```python
from build123d import *

# Parameters (mm, degrees)
F0_R      = 3
F0_R_2    = 2
F1_DEPTH  = 100
F2_R      = 3
F2_R_2    = 2
F3_DEPTH  = 6
F4_W      = 2
F4_H      = 7
F6_DEPTH  = 12.5
F5_W      = 2
F5_H      = 7
F7_DEPTH  = 12.5
F8_R      = 2
F9_DEPTH  = 34
F10_R     = 3.5
F10_R_2   = 3
F10_R_3   = 2
F11_DEPTH = 3


# Not quite as in the source:
# - a fillet or chamfer that OpenCascade refuses, or shapes differently, is made with other operations: its cross-section is extruded or revolved along the edge and cut away or added


with BuildPart() as f1:
    # F0 (on Top) → F1 (new body)
    with BuildSketch(Plane.XY):
        Circle(F0_R)
        Circle(F0_R_2, mode=Mode.SUBTRACT)
    extrude(amount=F1_DEPTH)

    # F2 (on face) → F3 (join)
    with BuildSketch(Plane.XY.offset(100)):
        Circle(F2_R)
        Circle(F2_R_2, mode=Mode.SUBTRACT)
        Circle(F2_R_2)
    extrude(amount=F3_DEPTH)

    # F4 (on Front) → F6 (cut, symmetric)
    with BuildSketch(Plane.XZ):
        with Locations((0, 85.1259604096)):
            Rectangle(F4_W, F4_H)
    extrude(amount=F6_DEPTH, both=True, mode=Mode.SUBTRACT)

    # F5 (on Right) → F7 (cut, symmetric)
    with BuildSketch(Plane.YZ):
        with Locations((0, 94.9563682079)):
            Rectangle(F5_W, F5_H)
    extrude(amount=F7_DEPTH, both=True, mode=Mode.SUBTRACT)

    # F8
    f8_edges = [f1.edges().sort_by_distance(p)[0] for p in [
        (-3, 0, 106),
    ]]
    fillet(f8_edges, radius=F8_R)

    # F9 (add): a face of the model
    f9_faces = [f1.faces().sort_by_distance(p)[0] for p in [
        (-2.9151471863, 0, 0),
    ]]
    extrude(f9_faces, amount=F9_DEPTH)

    # F10 (on face) → F11 (join)
    with BuildSketch(Plane(origin=(0, 0, -34), x_dir=(1, 0, 0), z_dir=(0, 0, -1))):
        Circle(F10_R)
        Circle(F10_R_2, mode=Mode.SUBTRACT)
        Circle(F10_R_2)
        Circle(F10_R_3, mode=Mode.SUBTRACT)
    extrude(amount=F11_DEPTH)

    # F12: fillet of radius 1 on 2 edges, made by hand

    # F12_s1 → F12_t2 (revolve, cut)
    with BuildSketch(Plane.XZ):
        with BuildLine():
            ThreePointArc((3, -34), (3.3660254038, -34.3660254038), (3.5, -34.8660254038))
            Line((3.5, -34.8660254038), (3.5, -34))
            Line((3.5, -34), (3, -34))
        make_face()
    revolve(axis=Axis((0, 0, -34), (0, 0, -1)), mode=Mode.SUBTRACT)

    # F12_s3 → F12_t4 (revolve, cut)
    with BuildSketch(Plane.XZ):
        with BuildLine():
            ThreePointArc((3.5, -36), (3.2071067812, -36.7071067812), (2.5, -37))
            Line((2.5, -37), (3.5, -37))
            Line((3.5, -37), (3.5, -36))
        make_face()
    revolve(axis=Axis((0, 0, -37), (0, 0, -1)), mode=Mode.SUBTRACT)


solid = f1.part
```
The model under review builds one solid part; all positions refer to its coordinate system, in mm. Round coordinates to 2 decimals unless told otherwise and drop trailing zeros. Loops run counter-clockwise (first coordinate to the right, second up) from the corner with the lowest first, then second, coordinate; pieces in that order, holes last. Notation, with made-up numbers: (78.25, 69.25) - (89.25, 69.25) arc R14 ccw to (89.25, 85.25) - close; hole circle Ø9 at (48, 51). An arc over 180 degrees is marked (long way). Use a Markdown table: item, result. Add a question column.
Q1. Add section B-B (z = 29.5). State the section outline as (x, y) points.
Q2. Add section A-A (z = 83.5). State the section outline as (x, y) points, plus the area to 3 significant figures.
Q3. The part is to be moulded in two halves that separate along X. For faces 1 (the face through (3.233, 1.341, -35.425)), 2 (the face through (0, 0, 100)), 3 (the face through (-1, -2, -37)), say which applies: pulls with the +X half, pulls with the -X half, needs draft (parallel to the pull), parting line crosses it, or undercut.
Q4. For probe 1 along X at (y, z) = (0, -35.55); probe 2 along Y at (x, z) = (0, 37.5); probe 3 along X at (y, z) = (1, 42), list the stretches that pass through material, from the lowest coordinate up.
Q5. Insertion check: pin 1 Ø1.2 at (y, z) = (2, 85.5) entering from +X; pin 2 Ø3.5 at (x, y) = (0, 0) entering from -Z; pin 3 Ø4 at (x, y) = (-2.5, -2.5) entering from -Z; pin 4 Ø0.5 at (x, z) = (2.5, 96) entering from -Y. Each pin has a flat end and moves straight along its axis. Give the tip position at first contact, or say it passes through.
Worked answers:
| question | item | result |
|---|---|---|
| 1 | outline | circle Ø6 at (0, 0); hole circle Ø4 at (0, 0) |
| 2 | outline | (-1, -2.83) - (-1, -1.73) arc R2 cw to (-1, 1.73) - (-1, 2.83) arc R3 ccw to start; (1, -2.83) arc R3 ccw to (1, 2.83) - (1, 1.73) arc R2 cw to (1, -1.73) - close |
| 2 | area | 11.6 mm² |
| 3 | face 1 | parting line crosses it |
| 3 | face 2 | undercut |
| 3 | face 3 | needs draft |
| 4 | probe 1 | -3.5 to -2, 2 to 3.5 |
| 4 | probe 2 | -3 to -2, 2 to 3 |
| 4 | probe 3 | -2.83 to -1.73, 1.73 to 2.83 |
| 5 | pin 1 | x = 2.65 |
| 5 | pin 2 | z = 100 |
| 5 | pin 3 | z = -37 |
| 5 | pin 4 | y = -1.98 |
